Geometry: final body of the model. Coordinates: model frame, mm. A direction names the side the tool comes from. Give positions to 0.01 mm unless a question says otherwise; leave off trailing zeros. Write each loop counter-clockwise with the first axis right and the second up, starting at its lowest first coordinate (ties: lowest second). Pieces come first, ordered by that corner, then holes. Notation, with made-up numbers: M 74.5,38.5 L 79.5,38.5 A23 ccw 79.5,62.5 Z; hole C 21.5,-31.75 d4. An arc over 180 degrees is marked long. Use one line per item in the form item = value. Start each with the question number.
Item 1: Section query B-B on z = 0.45. Return loops of the section in (x, y).
Item 2: Pull-direction query (X, two-part tool) for faces 3 (the flat face through (-2, 0, 6)), 4 (the flat face through (-7.03, 7.11, 2.96)), 5 (the flat face through (-2.3, 1.661, 5.5)); classes: released by +X, released by -X, zero draft, split by the parting line, or undercut.
Item 3: Section query C-C on y = 1. Return loops of the section in (x, z).
Item 4: Material intervals for line 1 along Y through (x, z) = (-5, 4.7); line 2 along Z through (x, y) = (-1, 2); line 3 along X through (y, z) = (4.25, 2.05), sorted ascending. Write a range as from..to.
Item 5: Section query A-A on z = 5.55. Return loops of the section in (x, y), then the cut area to 3 significant figures.
Item 6: Access query for faces 1 (the flat face through (1.74, 3.33, 5.51)), 2 (the flat face through (10, 0, 3)). Directions: +Z, -Z, +X, -X, +Y, -Y. A direction counts if a zero-diameter tool reaches every point of the face in a straight line with its end or side. Return the directions, or none.
Item 7: Section query D-D on x = 7.5. Return loops of the section in (y, z).
Item 8: Contact query for a flat-ended pin moving along its axis: P1, Ø1, axis at y = 5.5, z = 3.5, coming from the +X side. Output: stop coordinate, or through.
from build123d import *

# Parameters (mm, degrees)
F1_DEPTH = 6
F3_DEPTH = 1


with BuildPart() as f1:
    # F0 (on Top) → F1 (new body)
    with BuildSketch(Plane.XY):
        Polygon((10, -4.142136), (10, 4.142136), (4.142136, 10), (-4.142136, 10), (-10, 4.142136), (-10, -4.142136), (-4.142136, -10), (4.142136, -10), align=None)
    extrude(amount=F1_DEPTH)

    # F2 (on face) → F3 (cut)
    with BuildSketch(Plane.XY.offset(6)):
        Polygon((3.437641, 1.660818), (0, 5.046416), (-3.437641, 1.660818), (-1.204587, 1.660818), (-1.204587, -3.381562), (0, -3.381562), (1.204587, -3.381562), (1.204587, 1.660818), align=None)
    extrude(amount=-F3_DEPTH, mode=Mode.SUBTRACT)


solid = f1.part
Answer sheet:
q1.outline = M -10,-4.14 L -4.14,-10 L 4.14,-10 L 10,-4.14 L 10,4.14 L 4.14,10 L -4.14,10 L -10,4.14 Z
q2.face_3 = zero draft
q2.face_4 = released by -X
q2.face_5 = undercut
q3.outline = M -10,0 L 10,0 L 10,6 L 1.2,6 L 1.2,5 L -1.2,5 L -1.2,6 L -10,6 Z
q4.line_1 = -9.14..9.14
q4.line_2 = 0..5
q4.line_3 = -9.89..9.89
q5.outline = M -10,-4.14 L -4.14,-10 L 4.14,-10 L 10,-4.14 L 10,4.14 L 4.14,10 L -4.14,10 L -10,4.14 Z; hole M -3.44,1.66 L -1.2,1.66 L -1.2,-3.38 L 1.2,-3.38 L 1.2,1.66 L 3.44,1.66 L 0,5.05 Z
q5.area = 308 mm2
q6.face_1 = +Z
q6.face_2 = +Z, -Z, +X, +Y, -Y
q7.outline = M -6.64,0 L 6.64,0 L 6.64,6 L -6.64,6 Z
q8.P1 = 9.14
